Work out the finished part from the listing and answer in its coordinate system (mm). A direction names the side the tool comes from. Round coordinates to 2 decimals unless told otherwise and drop trailing zeros. Order: outer loops, then holes, each group sorted by start corner. A loop starts at its lowest first (then second) coordinate and runs counter-clockwise, first axis right, second up. Notation, with made-up numbers: (-13, 55) - (30, 55) arc R9 cw to (30, 60) - close; hole circle Ø8 at (14, -19). An arc over 180 degrees is marked (long way). Answer in a Markdown table with one row per item.
from build123d import *

# Parameters (mm, degrees)
F0_W     = 603.25
F0_H     = 609.6
F1_DEPTH = 304.8
F3_DEPTH = 304.8


with BuildPart() as f1:
    # F0 (on Front) → F1 (new body)
    with BuildSketch(Plane.XZ):
        with Locations((301.625, 304.8)):
            Rectangle(F0_W, F0_H)
        Polygon((283.766245, 304.8), (25.4, 43.464028), (25.4, 566.135972), align=None, mode=Mode.SUBTRACT)
        Polygon((559.991245, 25.4), (43.258755, 25.4), (301.625, 286.735972), align=None, mode=Mode.SUBTRACT)
        Polygon((577.85, 566.135972), (577.85, 42.503546), (319.008971, 304.319759), align=None, mode=Mode.SUBTRACT)
        Polygon((301.150216, 322.383787), (42.309187, 584.2), (559.991245, 584.2), align=None, mode=Mode.SUBTRACT)
    extrude(amount=F1_DEPTH)

    # F2 (on Front) → F3 (join)
    with BuildSketch(Plane.XZ):
        Polygon((12.7, 0), (0, 0), (0, -19.05), (25.4, -19.05), (25.4, -9.525), (12.7, -9.525), align=None)
        Polygon((80.9625, 0), (68.2625, 0), (68.2625, -9.525), (55.5625, -9.525), (55.5625, -19.05), (93.6625, -19.05), (93.6625, -9.525), (80.9625, -9.525), align=None)
        Polygon((149.225, 0), (136.525, 0), (136.525, -9.525), (123.825, -9.525), (123.825, -19.05), (161.925, -19.05), (161.925, -9.525), (149.225, -9.525), align=None)
        Polygon((217.4875, 0), (204.7875, 0), (204.7875, -9.525), (192.0875, -9.525), (192.0875, -19.05), (230.1875, -19.05), (230.1875, -9.525), (217.4875, -9.525), align=None)
        Polygon((411.1625, -19.05), (411.1625, -9.525), (398.4625, -9.525), (398.4625, 0), (385.7625, 0), (385.7625, -9.525), (373.0625, -9.525), (373.0625, -19.05), align=None)
        Polygon((479.425, -9.525), (466.725, -9.525), (466.725, 0), (454.025, 0), (454.025, -9.525), (441.325, -9.525), (441.325, -19.05), (479.425, -19.05), align=None)
        Polygon((547.6875, -9.525), (534.9875, -9.525), (534.9875, 0), (522.2875, 0), (522.2875, -9.525), (509.5875, -9.525), (509.5875, -19.05), (547.6875, -19.05), align=None)
        Polygon((603.25, 0), (590.55, 0), (590.55, -9.525), (577.85, -9.525), (577.85, -19.05), (603.25, -19.05), align=None)
    extrude(amount=F3_DEPTH)


solid = f1.part
1) The mould has two halves that part along X. Classify faces 3 (the face through (577.85, -150, 308)), 4 (the face through (0, -150, 300)), 5 (the face through (460, -150, -19.05)): released by +X, released by -X, zero draft, split by the parting line, or undercut.
Filled in:
| item | result |
|---|---|
| face 3 | undercut |
| face 4 | released by -X |
| face 5 | zero draft |
2) Find section B-B, the plane z = 182. Give the vertices of the cut face in (x, y), then the cut area to 3 significant figures.
Filled in:
| item | result |
|---|---|
| outline | (0, -304.8) - (25.4, -304.8) - (25.4, 0) - (0, 0) - close; (162.36, -304.8) - (198.08, -304.8) - (198.08, 0) - (162.36, 0) - close; (405.17, -304.8) - (439.94, -304.8) - (439.94, 0) - (405.17, 0) - close; (577.85, -304.8) - (603.25, -304.8) - (603.25, 0) - (577.85, 0) - close |
| area | 37,000 mm^2 |
3) Find the intervals of material crossed by probe 1 along X at (y, z) = (-68, 186.5); probe 2 along X at (y, z) = (-157.5, 421); probe 3 along Z at (x, y) = (326.5, -145), in increasing order. Write a range as from..to.
Filled in:
| item | result |
|---|---|
| probe 1 | x = 0..25.4, 166.81..202.53, 400.72..435.49, 577.85..603.25 |
| probe 2 | x = 0..25.4, 168.89..203.65, 398.65..434.36, 577.85..603.25 |
| probe 3 | z = 0..25.4, 261.58..296.74, 311.9..348.02, 584.2..609.6 |
4) Find section A-A, the plane x = 431.5. Give the vertices of the cut face in (y, z), then the cut area to 3 significant figures.
Filled in:
| item | result |
|---|---|
| outline | (-304.8, 0) - (0, 0) - (0, 25.4) - (-304.8, 25.4) - close; (-304.8, 155.37) - (0, 155.37) - (0, 190.54) - (-304.8, 190.54) - close; (-304.8, 418.1) - (0, 418.1) - (0, 454.23) - (-304.8, 454.23) - close; (-304.8, 584.2) - (0, 584.2) - (0, 609.6) - (-304.8, 609.6) - close |
| area | 37,200 mm^2 |
5) Find section C-C, the plane y = -120. Give the number of separate pieces and of enclosed holes in the cut face, then the cut area to 3 significant figures.
Filled in:
| item | result |
|---|---|
| separate pieces | 1 |
| enclosed holes | 4 |
| area | 101,000 mm^2 |
6) Which of the six approach directions +Z, -Z, +X, -X, +Y, -Y give full straight-line access (tool end or side, diameter ignored) to faces 1 (the face through (278, -304.8, 273)), 2 (the face through (429, -150.266, 157.897))?
Filled in:
| item | result |
|---|---|
| face 1 | +Z, -Z, +X, -X, -Y |
| face 2 | +Y, -Y |
7) This flat-tipped pin is pushed along its axis until it touches: pin 1 (16.5 mm diameter, centred on x = 179.5, y = -91, fed in from -Z). Where does it stop, or does it pass through?
Filled in:
| item | result |
|---|---|
| pin 1 | stops at z = 0 |
